Check sheet for the modelled part. Datum: model origin and axes. Units: mm. A direction names the side the tool comes from. Coordinates: 2 decimals unless noted, no trailing zeros. Write each loop counter-clockwise with the first axis right and the second up, starting at its lowest first coordinate (ties: lowest second). Pieces come first, ordered by that corner, then holes. Notation, with made-up numbers: (54, -17) -> (79, -17) arc R23 ccw to (79, 1) -> close; hole circle Ø10 at (12.25, -9.5). An arc over 180 degrees is marked (long way). One line per item, written item: value. Start each with the question number.
1) Set-up check for faces 4 (the cylindrical face through (-15.887, 4.645, 2.446)), 5 (the flat face through (-22, 27.66, 4)), 6 (the cylindrical face through (-32.906, 8.623, 3.767)): record each of +Z, -Z, +X, -X, +Y, -Y from which the full face is reachable in a straight line by a thin tool's end or side.
2) Gauge pin test, flat ends, axial feed: P1, Ø1, axis at x = -23.5, z = 3, coming from the +Y side; P2, Ø3, axis at y = 15, z = 5, coming from the +X side. Record the tip position at first contact, or that the pin passes through.
3) Draft check along Y on faces 1 (the cylindrical face through (-44.781, 15.537, 7.391)), 2 (the conical face through (-22.84, 4.45, 3.59)), 3 (the cylindrical face through (-37, 28.4, 3.8)). Enter one of: +Y half, -Y half, draft (parallel to the pull), parting line (faces both ways), or undercut.
4) Sectioned sample at A-A on x = -27.5. Enter the section's corners in (y, z), plus the area to 3 significant figures.
5) Scan lines: line 1 along Y through (x, z) = (-16, 3.81); line 2 along Y through (x, z) = (-29.5, 6.25); line 3 along Y through (x, z) = (-18, 4). Record each from-to range of solid material in increasing order. Write a range as [from, to].
```python
from build123d import *

# Parameters (mm, degrees)
F0_R     = 1.5875
F1_DEPTH = 7.62
F3_D     = 2.794
F3_DEPTH = 12.7
F3_TIP   = 0.8394022848
F5_D     = 2.794
F5_DEPTH = 12.7
F5_TIP   = 0.8394022848
F6_R     = 0.762
F7_R     = 0.762
F8_R     = 0.762


with BuildPart() as f1:
    # F0 (on Top) → F1 (new body)
    with BuildSketch(Plane.XY):
        with BuildLine():
            Line((-9.448561807, 27.6597626507), (-34.9631788839, 27.6597626507))
            ThreePointArc((-34.9631788839, 27.6597626507), (-37.027335895, 28.4223197326), (-38.0999731916, 30.3436959841))
            ThreePointArc((-38.0999731916, 30.3436959841), (-46.2053087095, 35.44162871), (-50.1456144211, 26.7146949509))
            Line((-50.1456144211, 26.7146949509), (-39.9539826805, 4.4896949509))
            ThreePointArc((-39.9539826805, 4.4896949509), (-37.6108431672, 1.7919340437), (-34.1819300664, 0.7865626507))
            Line((-34.1819300664, 0.7865626507), (-9.448561807, 0.7865626507))
            Line((-9.448561807, 0.7865626507), (-9.448561807, 7.8985626507))
            Line((-9.448561807, 7.8985626507), (-31.1296553504, 7.8985626507))
            ThreePointArc((-31.1296553504, 7.8985626507), (-32.9257065746, 8.6425114265), (-33.6696553504, 10.4385626507))
            Line((-33.6696553504, 10.4385626507), (-33.6696553504, 18.0077626507))
            ThreePointArc((-33.6696553504, 18.0077626507), (-32.9257065746, 19.8038138749), (-31.1296553504, 20.5477626507))
            Line((-31.1296553504, 20.5477626507), (-9.448561807, 20.5477626507))
            Line((-9.448561807, 20.5477626507), (-9.448561807, 27.6597626507))
        make_face()
        with Locations((-44.373561807, 29.3615626507)):
            Circle(F0_R, mode=Mode.SUBTRACT)
    extrude(amount=F1_DEPTH)

    # F3
    with Locations(Plane.YZ.offset(-9.448561807)):
        with Locations((24.1037626507, 3.81)):
            Hole(F3_D / 2, depth=F3_DEPTH)
            with Locations((0, 0, -(F3_DEPTH + F3_TIP / 2))):  # 118° drill point
                Cone(0, F3_D / 2, F3_TIP, mode=Mode.SUBTRACT)

    # F5
    with Locations(Plane.YZ.offset(-9.448561807)):
        with Locations((4.3425626507, 3.81)):
            Hole(F5_D / 2, depth=F5_DEPTH)
            with Locations((0, 0, -(F5_DEPTH + F5_TIP / 2))):  # 118° drill point
                Cone(0, F5_D / 2, F5_TIP, mode=Mode.SUBTRACT)

    # F6
    f6_edges = [f1.edges().sort_by_distance(p)[0] for p in [
        (-22.20587, 27.659763, 7.62),
    ]]
    fillet(f6_edges, radius=F6_R)

    # F7
    f7_edges = [f1.edges().sort_by_distance(p)[0] for p in [
        (-33.669655, 14.223163, 7.62),
    ]]
    fillet(f7_edges, radius=F7_R)

    # F8
    f8_edges = [f1.edges().sort_by_distance(p)[0] for p in [
        (-46.205309, 35.441629, 0),
        (-33.669655, 14.223163, 0),
    ]]
    fillet(f8_edges, radius=F8_R)


solid = f1.part
```
Answers:
1. face 4: +X
1. face 5: +Z, -Z, +X, +Y
1. face 6: +Z, -Z, +X
2. P1: stops at y = 27.66
2. P2: stops at x = -33.67
3. face 1: -Y half
3. face 2: undercut
3. face 3: +Y half
4. outline: (0.79, 0.76) arc R0.76 ccw to (1.55, 0) -> (7.14, 0) arc R0.76 ccw to (7.9, 0.76) -> (7.9, 6.86) arc R0.76 ccw to (7.14, 7.62) -> (1.55, 7.62) arc R0.76 ccw to (0.79, 6.86) -> close; (20.55, 0.76) arc R0.76 ccw to (21.31, 0) -> (26.9, 0) arc R0.76 ccw to (27.66, 0.76) -> (27.66, 6.86) arc R0.76 ccw to (26.9, 7.62) -> (21.31, 7.62) arc R0.76 ccw to (20.55, 6.86) -> close
4. area: 107 mm2
5. line 1: y = [0.79, 2.95], [5.74, 7.9], [20.55, 22.71], [25.5, 27.66]
5. line 2: y = [0.79, 7.9], [20.55, 27.66]
5. line 3: y = [0.79, 2.96], [5.73, 7.9], [20.55, 22.72], [25.49, 27.66]
